Autodesk Inventor part; units mm, degrees
ref_plane "YZ Plane" through (0, 0, 0) normal (1, 0, 0) x (0, 1, 0)
ref_plane "XZ Plane" through (0, 0, 0) normal (0, 1, 0) x (-1, 0, 0)
ref_plane "XY Plane" through (0, 0, 0) normal (0, 0, 1) x (1, 0, 0)
sketch "Sketch1" plane through (0, 0, 0) normal (0, 0, 1) x (1, 0, 0)
  line L0 (0, 0) -> (25.4, 0)
  line L1 (25.4, 0) -> (25.4, -50.8)
  line L2 (25.4, -50.8) -> (0, -50.8)
  line L3 (0, -50.8) -> (0, 0)
  line L4 (22.225, -3.175) -> (3.175, -3.175)
  line L5 (3.175, -3.175) -> (3.175, -47.625)
  line L6 (3.175, -47.625) -> (22.225, -47.625)
  line L7 (22.225, -47.625) -> (22.225, -3.175)
  dimension "d0" = 25.4
  dimension "d1" = 50.8
  dimension "d2" = 3.175
extrude "Extrusion1" add sketch "Sketch1" along normal blind 98.425
sketch "Sketch3" plane through (25.4, -50.8, 0) normal (1, 0, 0) x (0, 0, -1)
  circle A0 centre (-73.025, 25.4) radius 14.2875
  line L0 (0, 50.8) -> (-98.425, 50.8)
  line L1 (-98.425, 0) -> (-98.425, 50.8)
  dimension "d15" = 25.4
  dimension "d17" = 25.4
  dimension "d19" = 28.575
extrude "Extrusion3" cut sketch "Sketch3" against normal blind 38.1
properties part number "intake hinge"
The model under review builds one solid part; all positions refer to its coordinate system, in mm. A direction names the side the tool comes from. Give positions to 0.01 mm unless a question says otherwise; leave off trailing zeros. Order: outer loops, then holes, each group sorted by start corner. A loop starts at its lowest first (then second) coordinate and runs counter-clockwise, first axis right, second up. Notation, with made-up numbers: M 76,-12 L 104,-12 A19 ccw 104,15 Z; hole C 56.25,29.25 d8. An arc over 180 degrees is marked long. One line per question, with ' | ' between items. Start each with the question number.
1) Consider section A-A, the plane y = -46. Give the boundary of the cut face in (x, z) (3 decimals), then the cut area to 3 significant figures.
2) Mouldability with a two-part tool opening along X and no side actions: class faces 3 (the face through (2, -27, 98.425)), 4 (the face through (0, -26, 49)), 5 (the face through (25.4, -25, 49)), 6 (the face through (22.225, -26, 49)) as pulls with the +X half, pulls with the -X half, needs draft (parallel to the pull), parting line crosses it, or undercut.
3) Consider section B-B, the plane x = 2. Give the boundary of the cut face in (y, z) (1 decimal), then the cut area to 3 significant figures.
4) Wall thickness on L1, parallel to X at y = -29.5, z = 38 (3 decimals); L2, parallel to Y at x = 11.5, z = 18.5 (3 decimals); L3, parallel to Z at x = 24.75, y = -12.5 (3 decimals): over which ranges is each line inside the solid? List them lowest first. Write a range as from..to.
5) Consider section D-D, the plane z = 91.5. Give the boundary of the cut face in (x, y) (3 decimals).
6) Consider section C-C, the plane y = -25.4. Give the boundary of the cut face in (x, z) (1 decimal), then the cut area to 3 significant figures.
7) For faces 1 (the face through (13, -47.625, 49)), 2 (the face through (13, 0, 49)), list the 3-axis set-ups (+Z, -Z, +X, -X, +Y, -Y) from which the entire face can be reached by the end or side of a thin tool; tool diameter is ignored.
Found:
1) outline: M 0,0 L 3.175,0 L 3.175,98.425 L 0,98.425 Z; M 22.225,0 L 25.4,0 L 25.4,98.425 L 22.225,98.425 Z | area: 625 mm²
2) face 3: needs draft | face 4: pulls with the -X half | face 5: pulls with the +X half | face 6: undercut
3) outline: M -50.8,0 L 0,0 L 0,98.4 L -50.8,98.4 Z; hole C -25.4,73 d28.6 | area: 4,360 mm²
4) L1: x = 0..3.175, 22.225..25.4 | L2: y = -50.8..-47.625, -3.175..0 | L3: z = 0..66.883, 79.167..98.425
5) outline: M 0,-50.8 L 25.4,-50.8 L 25.4,0 L 0,0 Z; hole M 3.175,-47.625 L 22.225,-47.625 L 22.225,-3.175 L 3.175,-3.175 Z
6) outline: M 0,0 L 3.2,0 L 3.2,58.7 L 0,58.7 Z; M 0,87.3 L 3.2,87.3 L 3.2,98.4 L 0,98.4 Z; M 22.2,0 L 25.4,0 L 25.4,58.7 L 22.2,58.7 Z; M 22.2,87.3 L 25.4,87.3 L 25.4,98.4 L 22.2,98.4 Z | area: 444 mm²
7) face 1: +Z, -Z | face 2: +Z, -Z, +X, -X, +Y
